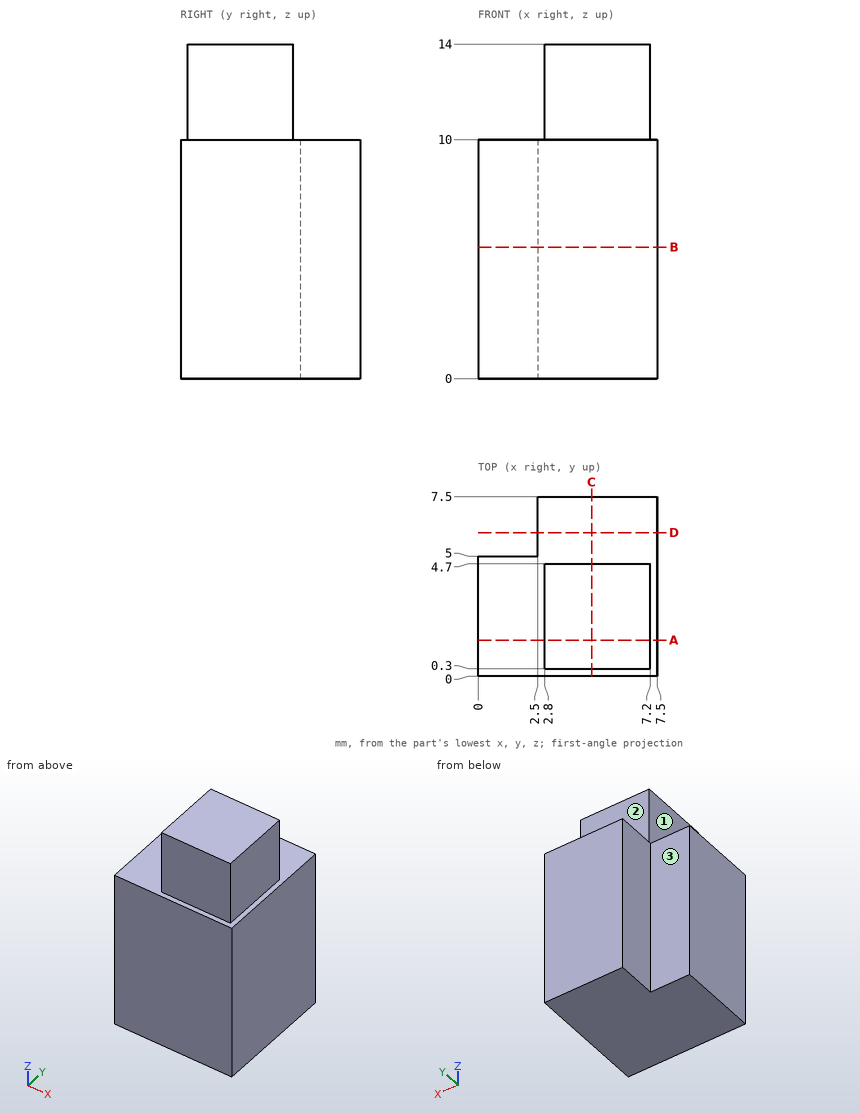
The figure shows three views and two pictorial views of one solid part (mm, origin at its lowest corner). Answer the questions. A direction names the side the tool comes from. Give positions to 0.01 mm unless a question says otherwise; leave off trailing zeros. Write each loop counter-clockwise with the first axis right and the second up, starting at its lowest first coordinate (ties: lowest second). Pieces come first, ordered by that corner, then holes. Notation, with made-up numbers: (-12.5, 78.5) -> (21.5, 78.5) arc R28 ccw to (21.5, 99.5) -> close; hole circle Ø1 at (-37.5, 25). An arc over 180 degrees is marked (long way). Use one line per item in the form item = value.
1) Section B-B on z = 5.5 is taken. Write down the section's boundary in (x, y).
Result:
outline = (0, 0) -> (7.5, 0) -> (7.5, 7.5) -> (2.5, 7.5) -> (2.5, 5) -> (0, 5) -> close
2) Section A-A on y = 1.5 is taken. Write down the section's boundary in (x, z).
Result:
outline = (0, 0) -> (7.5, 0) -> (7.5, 10) -> (7.2, 10) -> (7.2, 14) -> (2.8, 14) -> (2.8, 10) -> (0, 10) -> close
3) Straight lines are drawn through the part: probe 1 along Z at (x, y) = (3.5, 6.75); probe 2 along X at (y, z) = (6, 5.75); probe 3 along X at (y, z) = (2.5, 13.75). For each, find the intervals that lie inside material, in ascending order.
Result:
probe_1 = 0 to 10
probe_2 = 2.5 to 7.5
probe_3 = 2.8 to 7.2
4) Each of these flat-tipped pins is pushed along its axis until it touches: P1, Ø4.5, axis at y = 3, z = 12.5, coming from the -X side; P2, Ø0.8, axis at y = 5.5, z = 5, coming from the -X side; P3, Ø1.2, axis at x = 1, z = 7, coming from the +Y side. Where does it stop, or does it pass through?
Result:
P1 = 2.8
P2 = 2.5
P3 = 5
5) Section C-C on x = 4.75 is taken. Write down the section's boundary in (y, z), plus the area to 3 significant figures.
Result:
outline = (0, 0) -> (7.5, 0) -> (7.5, 10) -> (4.7, 10) -> (4.7, 14) -> (0.3, 14) -> (0.3, 10) -> (0, 10) -> close
area = 92.6 mm²
6) Section D-D on y = 6 is taken. Write down the section's boundary in (x, z), plus the area to 3 significant figures.
Result:
outline = (2.5, 0) -> (7.5, 0) -> (7.5, 10) -> (2.5, 10) -> close
area = 50.0 mm²
7) A tool of negligible diameter and unlimited length cuts with its end or side. For the marked faces 1, 2 and 3, from which of +Z, -Z, +X, -X, +Y, -Y can it reach the whole face along a straight path? Write none if from no direction.
Result:
face_1 = +Z, -X, +Y, -Y
face_2 = +Z, +X, -X, +Y
face_3 = +Z, -Z, -X, +Y
